Geometry check sheet. Reference: the model listing, model coordinates, mm. Face numbers are marked on the shaded views. A direction names the side the tool comes from. Round coordinates to 2 decimals unless told otherwise and drop trailing zeros. Order: outer loops, then holes, each group sorted by start corner. A loop starts at its lowest first (then second) coordinate and runs counter-clockwise, first axis right, second up. Notation, with made-up numbers: (54.25, -28) - (98.25, -28) arc R17 ccw to (98.25, -5) - close; hole circle Ø10 at (62.25, 13.25). An arc over 180 degrees is marked (long way). One line per question, with ' | ' between items. Start each with the question number.
Q1. Sectioned sample at B-B, the plane y = 0. Give the number of separate pieces and of enclosed holes in the cut face, then the cut area to 3 significant figures.
Q2. Material ranges on line 1 along Z through (x, y) = (80, -11.5); line 2 along X through (y, z) = (0, 34) (3 decimals), recorded low to high.
Q3. Gauge pin test, flat ends, axial feed: P1, Ø10, axis at x = -41.5, y = 9, coming from the -Z side; P2, Ø12, axis at y = 27, z = 24.5, coming from the -X side; P3, Ø15, axis at x = 54, z = -11.5, coming from the +Y side; P4, Ø1.5, axis at x = -93.5, z = -17, coming from the -Y side. Record the tip position at first contact, or that the pin passes through.
Q4. Sectioned sample at A-A, the plane x = -88.9. Enter the section's corners in (y, z) (3 decimals).
Q5. Mould release check, pull along Y, two halves, no side actions. Record for the marked faces 1, 2 and 3: +Y half, -Y half, draft (parallel to the pull), parting line (faces both ways), or undercut.
Q6. Tool access check on the marked faces 4, 5 and 6. Record the directions out of +Z, -Z, +X, -X, +Y, -Y that give a thin tool (end or side, any length) a straight path to the whole face; none if there is none.
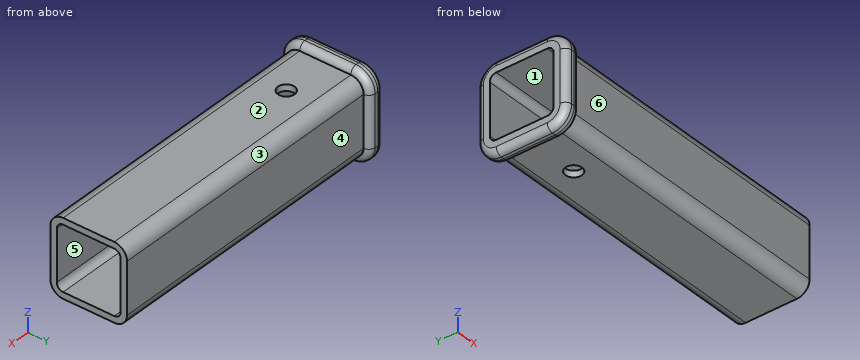
Autodesk Inventor part; units mm, degrees
ref_plane "YZ Plane" through (0, 0, 0) normal (1, 0, 0) x (0, 1, 0)
ref_plane "XZ Plane" through (0, 0, 0) normal (0, 1, 0) x (-1, 0, 0)
ref_plane "XY Plane" through (0, 0, 0) normal (0, 0, 1) x (1, 0, 0)
sketch "Sketch5" plane through (0, 0, 0) normal (1, 0, 0) x (0, 1, 0)
  line L0 (-25.4, 38.1) -> (25.4, 38.1)
  line L1 (38.1, 25.4) -> (38.1, -25.4)
  line L2 (25.4, -38.1) -> (-25.4, -38.1)
  line L3 (-38.1, -25.4) -> (-38.1, 25.4)
  line L4 (-38.1, 38.1) -> (38.1, -38.1) construction
  line L5 (38.1, 38.1) -> (-38.1, -38.1) construction
  arc A0 (38.1, 25.4) -> (25.4, 38.1) centre (25.4, 25.4) ccw
  arc A1 (25.4, -38.1) -> (38.1, -25.4) centre (25.4, -25.4) ccw
  arc A2 (-38.1, -25.4) -> (-25.4, -38.1) centre (-25.4, -25.4) ccw
  arc A3 (-25.4, 38.1) -> (-38.1, 25.4) centre (-25.4, 25.4) ccw
  line L6 (31.75, -25.4) -> (31.75, 25.4)
  arc A4 (31.75, 25.4) -> (25.4, 31.75) centre (25.4, 25.4) ccw
  line L7 (25.4, 31.75) -> (-25.4, 31.75)
  arc A5 (-25.4, 31.75) -> (-31.75, 25.4) centre (-25.4, 25.4) ccw
  line L8 (-31.75, 25.4) -> (-31.75, -25.4)
  arc A6 (-31.75, -25.4) -> (-25.4, -31.75) centre (-25.4, -25.4) ccw
  line L9 (-25.4, -31.75) -> (25.4, -31.75)
  arc A7 (25.4, -31.75) -> (31.75, -25.4) centre (25.4, -25.4) ccw
  point P0 (0, 0)
  dimension "d6" = 76.2
  dimension "d7" = 76.2
  dimension "d8" = 12.7
  dimension "d9" = 6.35
extrude "Extrusion4" add sketch "Sketch5" along normal mid plane 304.8
sketch "Sketch7" plane through (-152.4, 0, 0) normal (-1, 0, 0) x (0, 0, 1)
  arc A0 (-38.1, -25.4) -> (-25.4, -38.1) centre (-25.4, -25.4) ccw
  line L0 (-25.4, -38.1) -> (25.4, -38.1)
  arc A1 (25.4, -38.1) -> (38.1, -25.4) centre (25.4, -25.4) ccw
  line L1 (38.1, -25.4) -> (38.1, 25.4)
  arc A2 (38.1, 25.4) -> (25.4, 38.1) centre (25.4, 25.4) ccw
  line L2 (25.4, 38.1) -> (-25.4, 38.1)
  arc A3 (-25.4, 38.1) -> (-38.1, 25.4) centre (-25.4, 25.4) ccw
  line L3 (-38.1, 25.4) -> (-38.1, -25.4)
  arc A4 (-44.45, -25.4) -> (-25.4, -44.45) centre (-25.4, -25.4) ccw
  line L4 (-25.4, -44.45) -> (25.4, -44.45)
  arc A5 (25.4, -44.45) -> (44.45, -25.4) centre (25.4, -25.4) ccw
  line L5 (44.45, -25.4) -> (44.45, 25.4)
  arc A6 (44.45, 25.4) -> (25.4, 44.45) centre (25.4, 25.4) ccw
  line L6 (25.4, 44.45) -> (-25.4, 44.45)
  arc A7 (-25.4, 44.45) -> (-44.45, 25.4) centre (-25.4, 25.4) ccw
  line L7 (-44.45, 25.4) -> (-44.45, -25.4)
  point P0 (0, 0)
extrude "Extrusion5" add sketch "Sketch7" against normal blind 15.875
fillet "Fillet1" radius 6.35 16 edges at (-152.4, 38.8704, -38.8704) (-152.4, 0, -44.45) (-152.4, -38.8704, -38.8704) (-152.4, -44.45, 0) (-152.4, -38.8704, 38.8704) (-152.4, 0, 44.45) (-152.4, 38.8704, 38.8704) (-152.4, 44.45, 0) (-136.525, 38.8704, 38.8704) (-136.525, 0, 44.45) (-136.525, -38.8704, 38.8704) (-136.525, -44.45, 0) (-136.525, -38.8704, -38.8704) (-136.525, 0, -44.45) (-136.525, 38.8704, -38.8704) (-136.525, 44.45, 0)
sketch "Sketch8" plane through (0, 0, 0) normal (0, 0, 1) x (1, 0, 0)
  circle A0 centre (-88.9, 0) radius 8.255
  line L0 (-152.4, 25.4) -> (-152.4, -25.4)
  point P0 (0, 0)
  dimension "d15" = 63.5
  dimension "d16" = 16.51
extrude "Extrusion6" cut sketch "Sketch8" along normal through all both and the other way through all
properties part number "Model-1_Base Tube-3" material "SS304"
Determined:
1) separate pieces: 4 | enclosed holes: 0 | area: 3,830 mm2
2) line 1: z = -38.1 to -31.75, 31.75 to 38.1 | line 2: x = -152.4 to -97.155, -80.645 to 152.4
3) P1: stops at z = -38.1 | P2: stops at x = -152.4 | P3: stops at y = 38.1 | P4: stops at y = -38.1
4) outline: (-38.1, -25.4) arc R12.7 ccw to (-25.4, -38.1) - (-8.255, -38.1) - (-8.255, -31.75) - (-25.4, -31.75) arc R6.35 cw to (-31.75, -25.4) - (-31.75, 25.4) arc R6.35 cw to (-25.4, 31.75) - (-8.255, 31.75) - (-8.255, 38.1) - (-25.4, 38.1) arc R12.7 ccw to (-38.1, 25.4) - close; (8.255, -38.1) - (25.4, -38.1) arc R12.7 ccw to (38.1, -25.4) - (38.1, 25.4) arc R12.7 ccw to (25.4, 38.1) - (8.255, 38.1) - (8.255, 31.75) - (25.4, 31.75) arc R6.35 cw to (31.75, 25.4) - (31.75, -25.4) arc R6.35 cw to (25.4, -31.75) - (8.255, -31.75) - close
5) face 1: undercut | face 2: draft | face 3: +Y half
6) face 4: +Z, -Z, +X, +Y | face 5: +X, -X | face 6: +Z, -Z, +X, -Y
